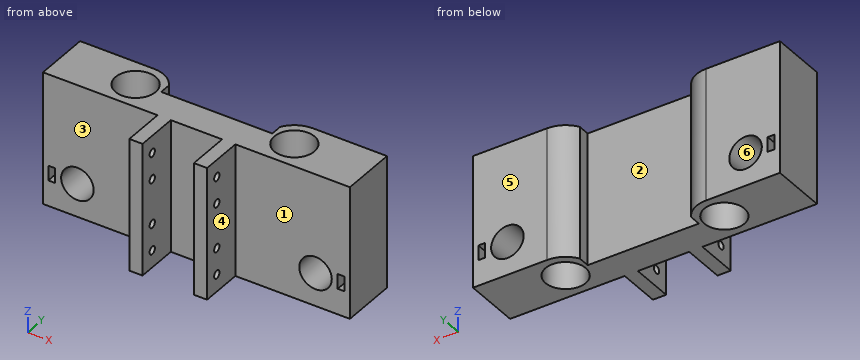
from build123d import *

# Parameters (mm, degrees)
SKETCH_R             = 7.6
PAD_DEPTH            = 50
SKETCH006_R          = 6.15
SKETCH006_W          = 2.6
SKETCH006_H          = 5.6
POCKET_DEPTH         = 10.501
POCKET_DEPTH_BACK    = 10.501
SKETCH015_W          = 42
SKETCH015_H          = 21
POCKET007_DEPTH      = 50.001
SKETCH022_W          = 5
SKETCH022_H          = 16
PAD010_DEPTH         = 50
SKETCH023_R          = 1.5
POCKET012_DEPTH      = 58.001
POCKET012_DEPTH_BACK = 58.001


with BuildPart() as part:
    # Sketch → Pad (new body)
    with BuildSketch(Plane.XY):
        with BuildLine():
            Line((-19.5477275198, 1), (19.5477275198, 1))
            ThreePointArc((30, 10.5), (22.9377765541, 7.770135134), (19.5477275198, 1))
            Line((58, 10.5), (30, 10.5))
            Line((58, -10.5), (58, 10.5))
            Line((58, -10.5), (-58, -10.5))
            Line((-58, -10.5), (-58, 10.5))
            Line((-58, 10.5), (-30, 10.5))
            ThreePointArc((-19.5477275198, 1), (-22.9377765541, 7.770135134), (-30, 10.5))
        make_face()
        with Locations((-30, 0)):
            Circle(SKETCH_R, mode=Mode.SUBTRACT)
        with Locations((30, 0)):
            Circle(SKETCH_R, mode=Mode.SUBTRACT)
    extrude(amount=PAD_DEPTH)

    # Sketch006 → Pocket (cut, two sides)
    with BuildSketch(Plane.XZ) as pocket_sk:
        with Locations((-45, 12.5)):
            Circle(SKETCH006_R)
        with Locations((45, 12.5)):
            Circle(SKETCH006_R)
        with Locations((-54.7, 12.5)):
            Rectangle(SKETCH006_W, SKETCH006_H)
        with Locations((54.7, 12.5)):
            Rectangle(SKETCH006_W, SKETCH006_H)
    extrude(amount=-POCKET_DEPTH, mode=Mode.SUBTRACT)
    extrude(pocket_sk.sketch, amount=POCKET_DEPTH_BACK, mode=Mode.SUBTRACT)

    # Sketch015 → Pocket007 (cut, through all)
    with BuildSketch(Plane.XY):
        with Locations((0, 11.5)):
            Rectangle(SKETCH015_W, SKETCH015_H)
    extrude(amount=POCKET007_DEPTH, mode=Mode.SUBTRACT)

    # Sketch022 → Pad010 (join)
    with BuildSketch(Plane.XY):
        with Locations((-12.2, -18.5)):
            Rectangle(SKETCH022_W, SKETCH022_H)
        with Locations((12.2, -18.5)):
            Rectangle(SKETCH022_W, SKETCH022_H)
    extrude(amount=PAD010_DEPTH)

    # Sketch023 → Pocket012 (cut, two sides)
    with BuildSketch(Plane.YZ) as pocket012_sk:
        with Locations((-21, 6.5)):
            Circle(SKETCH023_R)
        with Locations((-21, 16.5)):
            Circle(SKETCH023_R)
        with Locations((-21, 33.5)):
            Circle(SKETCH023_R)
        with Locations((-21, 43.5)):
            Circle(SKETCH023_R)
    extrude(amount=-POCKET012_DEPTH, mode=Mode.SUBTRACT)
    extrude(pocket012_sk.sketch, amount=POCKET012_DEPTH_BACK, mode=Mode.SUBTRACT)


with BuildPart() as part_1:
    # Body placement: moved
    add(part.part.moved(Location((0, 41, 0))))


solid = part_1.part
Check sheet for the modelled part. Datum: model origin and axes. Units: mm. Face numbers are marked on the shaded views. A direction names the side the tool comes from. Round coordinates to 2 decimals unless told otherwise and drop trailing zeros. Loops run counter-clockwise (first coordinate to the right, second up) from the corner with the lowest first, then second, coordinate; pieces in that order, holes last.
1. Sectioned sample at D-D on x = -27. Record the boundary of the cut face in (y, z).
2. Set-up check for the marked faces 1, 2 and 3: record each of +Z, -Z, +X, -X, +Y, -Y from which the full face is reachable in a straight line by a thin tool's end or side.
3. Sectioned sample at C-C on z = 12.5. Give the number of separate pieces and of enclosed holes in the cut face, and give its area (3 significant figures).
4. Scan lines: probe 1 along Z at (x, y) = (-11.5, 20); probe 2 along X at (y, z) = (48, 19.5); probe 3 along Y at (x, z) = (11, 33.5). Record each from-to range of solid material in increasing order.
5. Gauge pin test, flat ends, axial feed: pin 1 Ø5 at (x, z) = (24.5, 42) entering from -Y; pin 2 Ø4 at (y, z) = (20, 16.5) entering from -X; pin 3 Ø2.5 at (y, z) = (20, 33.5) entering from +X; pin 4 Ø5 at (y, z) = (23, 32.5) entering from +X. Record the tip position at first contact, or that the pin passes through.
6. Mould release check, pull along X, two halves, no side actions. Record for the marked faces 4, 5 and 6: released by +X, released by -X, zero draft, split by the parting line, or undercut.
7. Sectioned sample at B-B on x = -45. Record the boundary of the cut face in (y, z).
8. Sectioned sample at A-A on z = 43.5. Record the boundary of the cut face in (x, y).
Recorded:
1. outline: (30.5, 0) - (34.02, 0) - (34.02, 50) - (30.5, 50) - close; (47.98, 0) - (51.06, 0) - (51.06, 50) - (47.98, 50) - close
2. face 1: +Z, -Z, +X, -Y
2. face 2: +Z, -Z, +Y
2. face 3: +Z, -Z, -X, -Y
3. separate pieces: 5
3. enclosed holes: 2
3. area: 1,180 mm2
4. probe 1: z = 0 to 5, 8 to 15, 18 to 32, 35 to 42, 45 to 50
4. probe 2: x = -58 to -32.96, -27.04 to -22.17, 22.17 to 27.04, 32.96 to 58
4. probe 3: y = 14.5 to 18.5, 21.5 to 42
5. pin 1: stops at y = 30.5
5. pin 2: stops at x = -14.7
5. pin 3: passes through
5. pin 4: stops at x = 14.7
6. face 4: released by +X
6. face 5: zero draft
6. face 6: undercut
7. outline: (30.5, 0) - (51.5, 0) - (51.5, 6.35) - (30.5, 6.35) - close; (30.5, 18.65) - (51.5, 18.65) - (51.5, 50) - (30.5, 50) - close
8. outline: (-58, 30.5) - (-14.7, 30.5) - (-14.7, 21.5) - (-9.7, 21.5) - (-9.7, 30.5) - (9.7, 30.5) - (9.7, 21.5) - (14.7, 21.5) - (14.7, 30.5) - (58, 30.5) - (58, 51.5) - (30, 51.5) arc R10.5 ccw to (21, 46.41) - (21, 42) - (-21, 42) - (-21, 46.41) arc R10.5 ccw to (-30, 51.5) - (-58, 51.5) - close; (-14.7, 14.5) - (-9.7, 14.5) - (-9.7, 18.5) - (-14.7, 18.5) - close; (9.7, 14.5) - (14.7, 14.5) - (14.7, 18.5) - (9.7, 18.5) - close; hole circle Ø15.2 at (-30, 41); hole circle Ø15.2 at (30, 41)
